Check sheet for the modelled part. Datum: model origin and axes. Units: mm. A direction names the side the tool comes from. Coordinates: 2 decimals unless noted, no trailing zeros. Write each loop counter-clockwise with the first axis right and the second up, starting at its lowest first coordinate (ties: lowest second). Pieces come first, ordered by that corner, then holes. Notation, with made-up numbers: (68.5, 67) - (82.5, 67) arc R28 cw to (82.5, 97) - close; hole circle Ø9 at (28.25, -36). An arc over 180 degrees is marked (long way). Write each question's results on one line, items separated by ' | '.
from build123d import *

# Parameters (mm, degrees)
SKETCH3_R   = 11.1125
SKETCH3_8_R = 11.1125


with BuildPart() as part:
    # Sweep1: sweep along a path in Sketch1
    with BuildLine(Plane(origin=(0, 0, 0), x_dir=(0, 0, -1), z_dir=(1, 0, 0))) as sweep1_path:
        Line((0, -431.8), (152.212779539, -431.8))
        Line((152.212779539, -431.8), (584.012779539, -431.8))
        Line((584.012779539, -431.8), (584.012779539, -673.1))
        ThreePointArc((584.012779539, -673.1), (576.573291781, -691.060512242), (558.612779539, -698.5))
        Line((558.612779539, -698.5), (152.212779539, -698.5))
        Line((152.212779539, -698.5), (-0.187220461, -698.5))
    # Sketch3 → Sweep1 (sweep)
    with BuildSketch(Plane.XY):
        with Locations((0, -698.5)):
            Circle(SKETCH3_R)
    sweep(path=sweep1_path.line, transition=Transition.RIGHT)

    # Sweep2: sweep along a path in Sketch1<23>
    with BuildLine(Plane(origin=(0, 0, 0), x_dir=(0, 0, -1), z_dir=(1, 0, 0))) as sweep2_path:
        Line((-0.187220461, -698.5), (152.212779539, -698.5))
        Line((152.212779539, -698.5), (152.212779539, -431.8))
    # Sketch3<8> → Sweep2 (sweep)
    with BuildSketch(Plane.XY):
        with Locations((0, -698.5)):
            Circle(SKETCH3_8_R)
    sweep(path=sweep2_path.line, transition=Transition.RIGHT)


solid = part.part
1. Sectioned sample at C-C (y = -532). Record the cut outline in (x, z) (1 decimal), then the cut area to 3 significant figures.
Values follow:
outline: circle Ø22.2 at (0, -584); circle Ø22.2 at (0, -152.2) | area: 776 mm^2
2. Draft check along Z on faces 1 (the cylindrical face through (-2.41, -709.35, -275.3)), 2 (the flat face through (0, -432, 0)). Enter one of: pulls with the +Z half, pulls with the -Z half, needs draft (parallel to the pull), parting line crosses it, or undercut.
Values follow:
face 1: undercut | face 2: pulls with the +Z half
3. Access from +Z, -Z, +X, -X, +Y, -Y to the whole of each face (thin tool, end or side, straight path). Record for faces 3 (the cylindrical face through (-1.45, -563.28, -163.23)), 4 (the flat face through (0, -698, 0.187)).
Values follow:
face 3: none | face 4: +Z, +X, -X, +Y, -Y
4. Go/stop test with flat-tipped pins: pin 1 (11 mm diameter, centred on x = -1.5, y = -428.5, fed in from +Z); pin 2 (1 mm diameter, centred on x = -4.5, y = -524.5, fed in from -Z); pin 3 (8 mm diameter, centred on y = -450, z = -492.5, fed in from +X); pin 4 (3 mm diameter, centred on x = 4.5, z = -466.5, fed in from +Y). Record where each tip stops, or that it passes through.
Values follow:
pin 1: stops at z = 0 | pin 2: stops at z = -594.38 | pin 3: passes through | pin 4: stops at y = -421.1
5. Sectioned sample at B-B (z = -179). Record the cut outline in (x, y) (1 decimal).
Values follow:
outline: circle Ø22.2 at (0, -698.5); circle Ø22.2 at (0, -431.8)
6. Sectioned sample at A-A (x = 0). Record the cut outline in (y, z) (1 decimal).
Values follow:
outline: (-709.6, -558.6) arc R36.5 ccw to (-673.1, -595.1) - (-420.7, -595.1) - (-420.7, 0) - (-442.9, 0) - (-442.9, -141.1) - (-687.4, -141.1) - (-687.4, 0.2) - (-709.6, 0.2) - close; hole (-687.4, -558.6) arc R14.3 ccw to (-673.1, -572.9) - (-442.9, -572.9) - (-442.9, -163.3) - (-687.4, -163.3) - close
7. Material ranges on L1, parallel to Z at x = 1.25, y = -601; L2, parallel to Y at x = -0.75, z = -389; L3, parallel to Z at x = -5.75, y = -486.5, recorded low to high. Write a range as [from, to].
Values follow:
L1: z = [-595.05, -572.97], [-163.25, -141.17] | L2: y = [-709.59, -687.41], [-442.89, -420.71] | L3: z = [-593.52, -574.5], [-161.72, -142.7]
